```python
from build123d import *

# Parameters (mm, degrees)
SKETCH_1_R                       = 117.5
SKETCH_1_R_2                     = 90
EXTRUDE_1_DEPTH                  = 86
CHAMFER_1_SIZE                   = 3
SKETCH_2_R                       = 12.5
CUT_EXTRUDE_1_DEPTH              = 188.105585165
HOLE_WIZARD_M8_1_D               = 6.8
HOLE_WIZARD_M8_1_DEPTH           = 14
HOLE_WIZARD_M8_1_TIP             = 2.042926105
HOLE_WIZARD_M8_1_ON_FACE_2_D     = 6.8
HOLE_WIZARD_M8_1_ON_FACE_2_DEPTH = 14
HOLE_WIZARD_M8_1_ON_FACE_2_TIP   = 2.042926105
SCALE_1_SCALE                    = 0.2


with BuildPart() as part:
    # 草图1 → 凸台-拉伸1 (new body)
    with BuildSketch(Plane.XY):
        Circle(SKETCH_1_R)
        Circle(SKETCH_1_R_2, mode=Mode.SUBTRACT)
    extrude(amount=EXTRUDE_1_DEPTH)

    # 倒角1
    chamfer_1_edges = [part.edges().sort_by_distance(p)[0] for p in [
        (-117.5, 0, 0),
        (-117.5, 0, 86),
        (-90, 0, 0),
        (-90, 0, 86),
    ]]
    chamfer(chamfer_1_edges, length=CHAMFER_1_SIZE)

    # 草图2 → 切除-拉伸1 (cut, through all)
    with BuildSketch(Plane.XY.offset(86)):
        with Locations((0, 90)):
            Circle(SKETCH_2_R)
        with Locations((45, 77.942286341)):
            Circle(SKETCH_2_R)
        with Locations((77.942286341, 45)):
            Circle(SKETCH_2_R)
        with Locations((90, 0)):
            Circle(SKETCH_2_R)
        with Locations((77.942286341, -45)):
            Circle(SKETCH_2_R)
        with Locations((45, -77.942286341)):
            Circle(SKETCH_2_R)
        with Locations((0, -90)):
            Circle(SKETCH_2_R)
        with Locations((-45, -77.942286341)):
            Circle(SKETCH_2_R)
        with Locations((-77.942286341, -45)):
            Circle(SKETCH_2_R)
        with Locations((-90, 0)):
            Circle(SKETCH_2_R)
        with Locations((-77.942286341, 45)):
            Circle(SKETCH_2_R)
        with Locations((-45, 77.942286341)):
            Circle(SKETCH_2_R)
    extrude(amount=-CUT_EXTRUDE_1_DEPTH, mode=Mode.SUBTRACT)

    # M8 螺纹孔1
    with Locations(Plane(origin=(-25.88190451, 96.592582629, 86), x_dir=(1, 0, 0), z_dir=(0, 0, 1))):
        with Locations((0, 0), (96.592582629, -25.88190451), (-70.710678119, -70.710678119), (-44.828773609, -167.303260748), (51.76380902, -193.185165258), (122.474487139, -122.474487139)):
            Hole(HOLE_WIZARD_M8_1_D / 2, depth=HOLE_WIZARD_M8_1_DEPTH)
            with Locations((0, 0, -(HOLE_WIZARD_M8_1_DEPTH + HOLE_WIZARD_M8_1_TIP / 2))):  # 118° drill point
                Cone(0, HOLE_WIZARD_M8_1_D / 2, HOLE_WIZARD_M8_1_TIP, mode=Mode.SUBTRACT)

    # M8 螺纹孔1 on face 2
    with Locations(Plane(origin=(70.710678119, 70.710678119, 0), x_dir=(-1, 0, 0), z_dir=(0, 0, -1))):
        with Locations((0, 0), (96.592582629, 25.88190451), (167.303260748, -44.828773609), (141.421356238, -141.421356238), (44.828773609, -167.303260748), (-25.88190451, -96.592582629)):
            Hole(HOLE_WIZARD_M8_1_ON_FACE_2_D / 2, depth=HOLE_WIZARD_M8_1_ON_FACE_2_DEPTH)
            with Locations((0, 0, -(HOLE_WIZARD_M8_1_ON_FACE_2_DEPTH + HOLE_WIZARD_M8_1_ON_FACE_2_TIP / 2))):  # 118° drill point
                Cone(0, HOLE_WIZARD_M8_1_ON_FACE_2_D / 2, HOLE_WIZARD_M8_1_ON_FACE_2_TIP, mode=Mode.SUBTRACT)


with BuildPart() as part_1:
    # 缩放比例1: scaled about (0, 0, 0)
    add(part.part.scale(SCALE_1_SCALE))


solid = part_1.part
```
The listing builds one solid part. Answer for the finished solid, in the listing's coordinates (mm). A direction names the side the tool comes from. Give positions to 0.01 mm unless a question says otherwise; leave off trailing zeros. Write each loop counter-clockwise with the first axis right and the second up, starting at its lowest first coordinate (ties: lowest second). Pieces come first, ordered by that corner, then holes. Notation, with made-up numbers: (0, 37.5) - (44, 37.5) arc R24 ccw to (44, 58.5) - close; hole circle Ø11 at (17.5, 64). An arc over 180 degrees is marked (long way). Use one line per item in the form item = value. Start each with the question number.
1) Find section A-A on z = 4. Determine the outline of the cut face in (x, y).
2) Flat-ended cylindrical pins translate along their axes: pin 1 Ø6 at (y, z) = (10.5, 10) entering from -X; pin 2 Ø1.1 at (x, y) = (19.32, -5.18) entering from +Z; pin 3 Ø1.5 at (y, z) = (12.5, 11.5) entering from +X. Find the tip coordinate at first contact, or state that the pin passes through.
3) A tool of negligible diameter and unlimited length cuts with its end or side. For faces 1 (the face through (-5.324, 18.655, 1.42)), 2 (the face through (12.706, -12.75, 8.488)), 3 (the face through (4.77, 17.67, 16.9)), from which of +Z, -Z, +X, -X, +Y, -Y can it reach the whole face along a straight path? Write none if from no direction.
4) Consider line 1 along Y through (x, z) = (-13.5, 12.5); line 2 along X through (y, z) = (1.5, 7.5); line 3 along Y through (x, z) = (8.5, 8). Determine where each line is inside the solid, lowest interval first. Write a range as from..to.
Geometry results:
q1.outline = circle Ø47 at (0, 0); hole (-17.83, -2.49) arc R18 ccw to (-16.69, -6.75) arc R2.5 ccw (long way) to (-14.19, -11.07) arc R18 ccw to (-11.07, -14.19) arc R2.5 ccw (long way) to (-6.75, -16.69) arc R18 ccw to (-2.49, -17.83) arc R2.5 ccw (long way) to (2.49, -17.83) arc R18 ccw to (6.75, -16.69) arc R2.5 ccw (long way) to (11.07, -14.19) arc R18 ccw to (14.19, -11.07) arc R2.5 ccw (long way) to (16.69, -6.75) arc R18 ccw to (17.83, -2.49) arc R2.5 ccw (long way) to (17.83, 2.49) arc R18 ccw to (16.69, 6.75) arc R2.5 ccw (long way) to (14.19, 11.07) arc R18 ccw to (11.07, 14.19) arc R2.5 ccw (long way) to (6.75, 16.69) arc R18 ccw to (2.49, 17.83) arc R2.5 ccw (long way) to (-2.49, 17.83) arc R18 ccw to (-6.75, 16.69) arc R2.5 ccw (long way) to (-11.07, 14.19) arc R18 ccw to (-14.19, 11.07) arc R2.5 ccw (long way) to (-16.69, 6.75) arc R18 ccw to (-17.83, 2.49) arc R2.5 ccw (long way) to start
q2.pin_1 = -22.27
q2.pin_2 = 14.32
q2.pin_3 = 20.35
q3.face_1 = -Z
q3.face_2 = +Z, -Z
q3.face_3 = +Z
q4.line_1 = -19.24..-11.91, 11.91..19.24
q4.line_2 = -23.45..-20, 20..23.45
q4.line_3 = -21.91..-18.04, 18.04..21.91
